```python
from build123d import *

# Parameters (mm, degrees)
F0_W     = 45
F0_H     = 16.3
F1_DEPTH = 15
F3_DEPTH = 12
F4_W     = 45
F4_H     = 15
F5_DEPTH = 1
F6_W     = 45
F6_H     = 15
F7_DEPTH = 1


with BuildPart() as f1:
    # F0 (on Top) → F1 (new body)
    with BuildSketch(Plane.XY):
        Rectangle(F0_W, F0_H)
    extrude(amount=F1_DEPTH)

    # F2 (on face) → F3 (cut)
    with BuildSketch(Plane.XY.offset(15)):
        Polygon((-21, -5.85), (-21, -6.15), (-17.5, -6.15), (-17.5, -8.15), (12.5, -8.15), (12.5, -6.15), (21, -6.15), (21, -5.85), (12.5, -5.85), (12.5, -3.15), (21, -3.15), (21, -2.85), (12.5, -2.85), (12.5, -0.15), (21, -0.15), (21, 0.15), (12.5, 0.15), (12.5, 2.85), (21, 2.85), (21, 3.15), (12.5, 3.15), (12.5, 5.85), (21, 5.85), (21, 6.15), (12.5, 6.15), (12.5, 8.15), (-17.5, 8.15), (-17.5, 6.15), (-21, 6.15), (-21, 5.85), (-17.5, 5.85), (-17.5, 3.15), (-21, 3.15), (-21, 2.85), (-17.5, 2.85), (-17.5, 0.15), (-21, 0.15), (-21, -0.15), (-17.5, -0.15), (-17.5, -2.85), (-21, -2.85), (-21, -3.15), (-17.5, -3.15), (-17.5, -5.85), align=None)
    extrude(amount=-F3_DEPTH, mode=Mode.SUBTRACT)

    # F4 (on face) → F5 (join)
    with BuildSketch(Plane.XZ.offset(8.15)):
        with Locations((0, 7.5)):
            Rectangle(F4_W, F4_H)
    extrude(amount=F5_DEPTH)

    # F6 (on face) → F7 (join)
    with BuildSketch(Plane(origin=(0, 8.15, 0), x_dir=(-1, 0, 0), z_dir=(0, 1, 0))):
        with Locations((0, 7.5)):
            Rectangle(F6_W, F6_H)
    extrude(amount=F7_DEPTH)


solid = f1.part
```
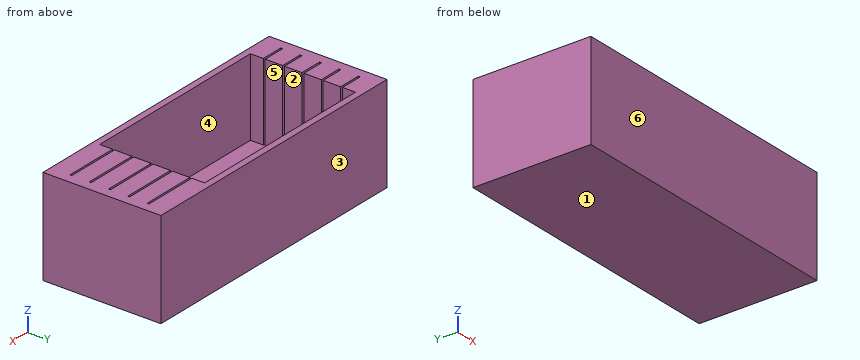
The model under review builds one solid part; all positions refer to its coordinate system, in mm. Face numbers are marked on the shaded views. A direction names the side the tool comes from. Coordinates: 2 decimals unless noted, no trailing zeros. Write each loop counter-clockwise with the first axis right and the second up, starting at its lowest first coordinate (ties: lowest second). Pieces come first, ordered by that corner, then holes. Notation, with made-up numbers: (-35, 1.5) -> (17, 1.5) arc R29 cw to (17, 29.5) -> close; hole circle Ø7 at (56.5, 25.25). An arc over 180 degrees is marked (long way). One line per item, written item: value. Start each with the question number.
Q1. The part is to be moulded in two halves that separate along Y. For the marked faces 1, 2, 3 and 4, say which applies: +Y half, -Y half, draft (parallel to the pull), parting line (faces both ways), or undercut.
Q2. Add section C-C, the plane x = 17. Give the boundary of the cut face in (y, z), then the cut area to 4 significant figures.
Q3. For the marked faces 5 and 6, list the 3-axis set-ups (+Z, -Z, +X, -X, +Y, -Y) from which the entire face can be reached by the end or side of a thin tool; tool diameter is ignored.
Q4. To check wall thickness, follow probe 1 along Y at (x, z) = (19, 10); probe 2 along X at (y, z) = (5, 13); probe 3 along Y at (x, z) = (4.5, 6.75). State the ranges of each line that lie inside material, in increasing order.
Q5. Add section B-B, the plane y = -3.75. Give the boundary of the cut face in (x, z).
Q6. Add section A-A, the plane x = -7. Give the boundary of the cut face in (y, z).
Response:
1. face 1: draft
1. face 2: undercut
1. face 3: +Y half
1. face 4: undercut
2. outline: (-9.15, 0) -> (9.15, 0) -> (9.15, 15) -> (6.15, 15) -> (6.15, 3) -> (5.85, 3) -> (5.85, 15) -> (3.15, 15) -> (3.15, 3) -> (2.85, 3) -> (2.85, 15) -> (0.15, 15) -> (0.15, 3) -> (-0.15, 3) -> (-0.15, 15) -> (-2.85, 15) -> (-2.85, 3) -> (-3.15, 3) -> (-3.15, 15) -> (-5.85, 15) -> (-5.85, 3) -> (-6.15, 3) -> (-6.15, 15) -> (-9.15, 15) -> close
2. area: 256.5 mm²
3. face 5: +Z
3. face 6: +Z, -Z, +X, -X, -Y
4. probe 1: -9.15 to -6.15, -5.85 to -3.15, -2.85 to -0.15, 0.15 to 2.85, 3.15 to 5.85, 6.15 to 9.15
4. probe 2: -22.5 to -17.5, 12.5 to 22.5
4. probe 3: -9.15 to -8.15, 8.15 to 9.15
5. outline: (-22.5, 0) -> (22.5, 0) -> (22.5, 15) -> (12.5, 15) -> (12.5, 3) -> (-17.5, 3) -> (-17.5, 15) -> (-22.5, 15) -> close
6. outline: (-9.15, 0) -> (9.15, 0) -> (9.15, 15) -> (8.15, 15) -> (8.15, 3) -> (-8.15, 3) -> (-8.15, 15) -> (-9.15, 15) -> close
